Autodesk Inventor part; units mm, degrees
ref_plane "YZ Plane" through (0, 0, 0) normal (1, 0, 0) x (0, 1, 0)
ref_plane "XY Plane" through (0, 0, 0) normal (0, 0, 1) x (1, 0, 0)
sketch "Sketch1" plane through (0, 0, 0) normal (1, 0, 0) x (0, 1, 0)
  arc A0 (1.1581, -1.06) -> (-1.1581, -1.06) centre (0, 0) ccw
  line L0 (1.1581, -1.06) -> (-1.1581, -1.06)
  circle A1 centre (0, 0) radius 26.5
extrude "Extrusion1" add sketch "Sketch1" along normal blind 10
ref_plane "Work Plane1" through (0, 26.5, 0) normal (0, 1, 0) x (-1, 0, 0)
ref_plane "Work Plane2" through (0, -26.5, 0) normal (0, 1, 0) x (-1, 0, 0)
sketch "Sketch6" plane through (10, 0, 0) normal (1, 0, 0) x (0, 0, -1)
  arc A0 (26.4953, 0.5) -> (26.4953, -0.5) centre (0, 0) ccw
  line L0 (0, 26.5) -> (0, 27.25)
  arc A1 (26.4953, 0.5) -> (26.4953, -0.5) centre (0, 0) ccw
  circle A2 centre (0, 0) radius 26.5
  circle A3 centre (0, 0) radius 26.5
  circle A4 centre (0, 0) radius 27.25
  dimension "d22" = 0.75
extrude "Extrusion6" add sketch "Sketch6" against normal blind 1
ref_plane "Work Plane3" through (5, 0, 0) normal (1, 0, 0) x (0, 0, -1)
mirror "Mirror1" about plane through (5, 0, 0) normal (1, 0, 0) of "Extrusion6"
sketch "Sketch7" plane through (0, -1.1581, -1.06) normal (0, 0, 1) x (1, 0, 0)
  line L0 (1, 27.6581) -> (9, 27.6581)
  line L1 (5, 27.6581) -> (5, -25.3419)
  line L2 (1, -25.3419) -> (9, -25.3419)
  line L3 (10, 2.3163) -> (10, 0)
  line L4 (10, 1.1581) -> (-0.1429, 1.1581)
  circle A0 centre (5, 1.1581) radius 1.8
  dimension "d28" = 3.6
extrude "Extrusion7" cut sketch "Sketch7" against normal blind 13
ref_plane "Work Plane4" through (10, -1.1581, -14.06) normal (0, 0, 1) x (1, 0, 0)
sketch "Sketch8" plane through (10, -1.1581, -14.06) normal (0, 0, 1) x (1, 0, 0)
  arc A0 (-6.3779, 0) -> (-3.6221, 0) centre (-5, 1.1581) ccw
  circle A1 centre (-5, 1.1581) radius 2.05
  point P0 (-10, 1.1581)
  dimension "d32" = 4.1
extrude "Extrusion8" cut sketch "Sketch8" against normal blind 6
ref_plane "Work Plane5" through (10, -1.1581, -20.06) normal (0, 0, 1) x (1, 0, 0)
sketch "Sketch10" plane through (10, 0, 0) normal (1, 0, 0) x (0, 0, -1)
  circle A0 centre (0, 0) radius 27.25
  circle A1 centre (0, 0) radius 1.75
  line L0 (1.2405, 1.2351) -> (1.2405, -1.2351)
  arc A2 (1.2405, 1.2351) -> (1.2405, -1.2351) centre (0, 0) ccw
  point P0 (1.2405, -1.2344)
  point P1 (1.2405, 1.2344)
  dimension "d40" = 3.5
extrude "Extrusion10" cut sketch "Sketch10" against normal blind 15.575 contours L0 A1 picked at (0.3435, -0.5243)
sketch "Sketch11" plane through (10, 0, 0) normal (1, 0, 0) x (0, 0, -1)
  circle A0 centre (0, 0) radius 27.25
  arc A1 (1.2405, 1.2344) -> (1.2405, -1.2344) centre (0, 0) ccw
  circle A2 centre (0, 0) radius 25.4
  dimension "d44" = 50.8
extrude "Extrusion11" cut sketch "Sketch11" against normal blind 10
sketch "Sketch12" plane through (5, 0, 0) normal (1, 0, 0) x (0, 0, -1)
  circle A0 centre (0, 0) radius 28
  circle A1 centre (0, 0) radius 25.4
  dimension "d45" = 56
extrude "Extrusion12" add sketch "Sketch12" along normal mid plane 5
sketch "Sketch9" plane through (10, -1.1581, -20.06) normal (0, 0, 1) x (1, 0, 0)
  circle A0 centre (-5, 1.1581) radius 1.8
  circle A1 centre (-5, 1.1581) radius 4.3333
  circle A2 centre (-5, 1.1581) radius 2.05
  circle A3 centre (-5, 1.1581) radius 3.25
  point P0 (-10, 1.1581)
  dimension "d41" = 6.5
extrude "Extrusion9" cut sketch "Sketch9" against normal blind 16.225 contours A0 | A2 | A3
fillet "Fillet1" radius 2 4 edges at (2.5, 2.0767, -26.6189) (2.5, -2.0767, -26.6189) (7.5, -2.0767, -26.6189) (7.5, 2.0767, -26.6189)
properties part number "Lock Wheel New Rubber"
Source: CAD feature listing. Evaluate the final solid. Frame: model axes, mm. A direction names the side the tool comes from. Give positions to 0.01 mm unless a question says otherwise; leave off trailing zeros. Order: outer loops, then holes, each group sorted by start corner. A loop starts at its lowest first (then second) coordinate and runs counter-clockwise, first axis right, second up. Notation, with made-up numbers: (-2.75, -25.75) -> (53.25, -25.75) arc R32 cw to (53.25, 6.25) -> close; hole circle Ø11 at (-31, 9). An arc over 180 degrees is marked (long way). Write item = value, one per line.
Q1. Material intervals for line 1 (X direction, y = 0, z = -22); line 2 (Y direction, x = 5, z = 0); line 3 (X direction, y = 0, z = -9), sorted ascending. Write a range as from..to.
Data:
line_1 = 0..1.75, 8.25..10
line_2 = -28..-1.75, 1.75..28
line_3 = 0..3.2, 6.8..10
Q2. Cut plane C-C, the plane x = 1. Output: boundary loops of the cut face in (y, z), and give its area (3 significant figures).
Data:
outline = circle Ø50.8 at (0, 0); hole (-1.24, -1.24) -> (1.24, -1.24) arc R1.75 ccw (long way) to start
area = 2,020 mm^2
Q3. Cut plane A-A, the plane z = 0. Output: boundary loops of the cut face in (x, y), and give its area (3 significant figures).
Data:
outline = (0, -25.4) -> (2.5, -25.4) -> (2.5, -28) -> (7.5, -28) -> (7.5, -25.4) -> (10, -25.4) -> (10, -1.75) -> (0, -1.75) -> close; (0, 1.75) -> (10, 1.75) -> (10, 25.4) -> (7.5, 25.4) -> (7.5, 28) -> (2.5, 28) -> (2.5, 25.4) -> (0, 25.4) -> close
area = 499 mm^2
Q4. Pull-direction query (Z, two-part tool) for faces 5 (the face through (1.336, -22.534, -11.721)), 6 (the face through (2, 0, -1.24)), 7 (the face through (8, 0, -1.24)), 8 (the face through (6.717, 0.541, -7.469)); classes: released by +Z, released by -Z, zero draft, split by the parting line, or undercut.
Data:
face_5 = split by the parting line
face_6 = undercut
face_7 = undercut
face_8 = zero draft
Q5. Pin query (flat end, axial travel): pin 1 (2 mm diameter, centred on x = 3, z = -9.5, fed in from +Y); pin 2 (2 mm diameter, centred on x = 9, y = 0, fed in from +Z); pin 3 (3.5 mm diameter, centred on x = 5, y = 0, fed in from +Z); pin 4 (2 mm diameter, centred on y = 0, z = 0, fed in from +X). Return the tip coordinate at first contact, or that it passes through.
Data:
pin_1 = 26.68
pin_2 = 25.4
pin_3 = 28
pin_4 = through
Q6. Set-up query: faces 1 (the face through (2.5, -6, 25)), 2 (the face through (5.07, 0.06, 1.75)), 3 (the face through (6, -2, -20.06)), 4 (the face through (8.73, 7.629, -24.227)). Return all of +Z, -Z, +X, -X, +Y, -Y with unobstructed straight access to the full face (end or side cutting, diameter ignored); none if empty.
Data:
face_1 = -X
face_2 = +X, -X
face_3 = -Z
face_4 = +X
Q7. Cut plane B-B, the plane y = 0. Output: boundary loops of the cut face in (x, z).
Data:
outline = (0, -25.4) -> (1.75, -25.4) -> (1.75, -20.06) -> (2.95, -20.06) -> (2.95, -14.06) -> (3.2, -14.06) -> (3.2, -1.24) -> (0, -1.24) -> close; (0, 1.75) -> (10, 1.75) -> (10, 25.4) -> (7.5, 25.4) -> (7.5, 28) -> (2.5, 28) -> (2.5, 25.4) -> (0, 25.4) -> close; (6.8, -14.06) -> (7.05, -14.06) -> (7.05, -20.06) -> (8.25, -20.06) -> (8.25, -25.4) -> (10, -25.4) -> (10, -1.24) -> (6.8, -1.24) -> close
Q8. Cut plane D-D, the plane z = 12.5. Output: boundary loops of the cut face in (x, y), and give its area (3 significant figures).
Data:
outline = (0, -22.11) -> (2.5, -22.11) -> (2.5, -25.05) -> (7.5, -25.05) -> (7.5, -22.11) -> (10, -22.11) -> (10, 22.11) -> (7.5, 22.11) -> (7.5, 25.05) -> (2.5, 25.05) -> (2.5, 22.11) -> (0, 22.11) -> close
area = 472 mm^2
